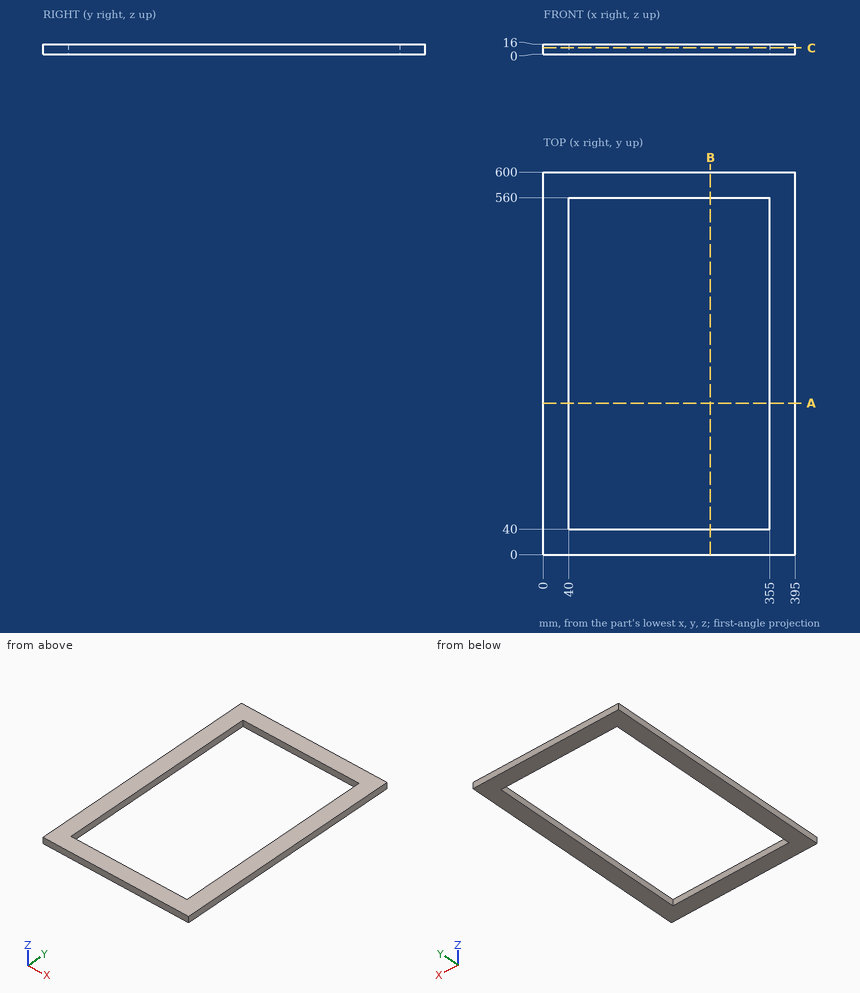
Design review of the part shown in the three views and the two pictorial views. Dimensions are in mm from the part's minimum x, y and z. Coordinates: 2 decimals unless noted, no trailing zeros. Loops run counter-clockwise (first coordinate to the right, second up) from the corner with the lowest first, then second, coordinate; pieces in that order, holes last.
Q1. To check wall thickness, follow line 1 (X direction, y = 448, z = 2.5); line 2 (Y direction, x = 143, z = 3). State the ranges of each line that lie inside material, in increasing order.
Reported:
line 1: x = 0 to 40, 355 to 395
line 2: y = 0 to 40, 560 to 600
Q2. We need section A-A on y = 237.5. State the section outline as (x, z) points, and give its area (3 significant figures).
Reported:
outline: (0, 0) - (40, 0) - (40, 16) - (0, 16) - close; (355, 0) - (395, 0) - (395, 16) - (355, 16) - close
area: 1,280 mm2
Q3. We need section C-C on z = 9.75. State the section outline as (x, y) points, and give its area (3 significant figures).
Reported:
outline: (0, 0) - (395, 0) - (395, 600) - (0, 600) - close; hole (40, 40) - (355, 40) - (355, 560) - (40, 560) - close
area: 73,200 mm2
Q4. We need section B-B on x = 262. State the section outline as (y, z) points.
Reported:
outline: (0, 0) - (40, 0) - (40, 16) - (0, 16) - close; (560, 0) - (600, 0) - (600, 16) - (560, 16) - close
Q5. For pin 1 (5 mm diameter, centred on x = 159, z = 7.5, fed in from -Y), flat-tipped, find the tip position at first contact; note if it passes through.
Reported:
pin 1: stops at y = 0
